Design review of the part built by this model. Coordinates are the model's own, in mm. Face numbers are marked on the shaded views. A direction names the side the tool comes from. Give positions to 0.01 mm unless a question says otherwise; leave off trailing zeros. Loops run counter-clockwise (first coordinate to the right, second up) from the corner with the lowest first, then second, coordinate; pieces in that order, holes last. Notation, with made-up numbers: (63, -16) -> (87, -16) arc R32 ccw to (87, 16) -> close; hole circle Ø10 at (-18, 18.25). An arc over 180 degrees is marked (long way). Answer in a Markdown table with one row per item. Add a question column.
(1) Consider section B-B on x = 12.5. Write out the cut boundary in (y, z), then the cut area to 3 significant figures.
(2) Draft analysis for pull direction Y (two halves, no side actions). For the marked faces 1, 2 and 3, state which applies: +Y half, -Y half, draft (parallel to the pull), parting line (faces both ways), or undercut.
(3) For line 1 (X direction, y = 25.5, z = -0.4); line 2 (Y direction, x = -12.5, z = 1.3); line 3 (X direction, y = -17.5, z = -0.25), list the stretches that pass through material, from the lowest coordinate up.
(4) Consider section D-D on y = 1.5. Write out the cut boundary in (x, z), then the cut area to 3 significant figures.
(5) For pin 1 (5 mm diameter, centred on x = -12.5, y = -12.5, fed in from -Z); pin 2 (2 mm diameter, centred on x = -2.5, z = 2, fed in from +Y); pin 3 (1.5 mm diameter, centred on y = 4.5, z = 2.5, fed in from -X), all flat-tipped, find the tip position at first contact; note any pin that passes through.
(6) Consider section A-A on x = -0.5. Write out the cut boundary in (y, z).
(7) For the marked faces 4 and 5, list the 3-axis set-ups (+Z, -Z, +X, -X, +Y, -Y) from which the entire face can be reached by the end or side of a thin tool; tool diameter is ignored.
(8) Consider section C-C on z = -3.25. Write out the cut boundary in (x, y).
from build123d import *

# Parameters (mm, degrees)
F0_R     = 1.6
F0_W     = 12
F0_H     = 15
F1_DEPTH = 4
F2_R     = 2.25
F3_DEPTH = 1
F4_DEPTH = 5
F5_R     = 5


# Not quite as in the source:
# - ends of sketch curves that miss each other by under 0.0002 mm in the source are joined


with BuildPart() as f1:
    # F0 (on Top) → F1 (new body)
    with BuildSketch(Plane.XY):
        Polygon((-26.600003, -29.899997), (-26.5, -30), (-10, -30), (10, -30), (26.5, -30), (26.6, -29.9), (27, -29.5), (27, -13), (27, 13), (27, 29.5), (26.5999975, 29.9000025), (26.5, 30), (10, 30), (-10, 30), (-26.5, 30), (-26.599999, 29.900001), (-27, 29.5), (-27, 13), (-27, -13), (-27, -29.5), align=None)
        with BuildLine():
            ThreePointArc((-22.5, -23.25), (-20.9090097423, -23.9090097423), (-20.25, -25.5))
            ThreePointArc((-20.25, -25.5), (-20.9090097423, -27.0909902577), (-22.5, -27.75))
            ThreePointArc((-22.5, -27.75), (-24.0909902577, -27.0909902577), (-24.75, -25.5))
            ThreePointArc((-24.75, -25.5), (-24.0909902577, -23.9090097423), (-22.5, -23.25))
        make_face(mode=Mode.SUBTRACT)
        with Locations((-12.5, -12.5)):
            Circle(F0_R, mode=Mode.SUBTRACT)
        with BuildLine():
            ThreePointArc((22.5, -23.25), (24.0909902577, -23.9090097423), (24.75, -25.5))
            ThreePointArc((24.75, -25.5), (24.0909902577, -27.0909902577), (22.5, -27.75))
            ThreePointArc((22.5, -27.75), (20.9090097423, -27.0909902577), (20.25, -25.5))
            ThreePointArc((20.25, -25.5), (20.9090097423, -23.9090097423), (22.5, -23.25))
        make_face(mode=Mode.SUBTRACT)
        with Locations((12.5, -12.5)):
            Circle(F0_R, mode=Mode.SUBTRACT)
        with Locations((-12.5, 12.5)):
            Circle(F0_R, mode=Mode.SUBTRACT)
        with BuildLine():
            ThreePointArc((-22.5, 27.75), (-20.9090097423, 27.0909902577), (-20.25, 25.5))
            ThreePointArc((-20.25, 25.5), (-20.9090097423, 23.9090097423), (-22.5, 23.25))
            ThreePointArc((-22.5, 23.25), (-24.0909902577, 23.9090097423), (-24.75, 25.5))
            ThreePointArc((-24.75, 25.5), (-24.0909902577, 27.0909902577), (-22.5, 27.75))
        make_face(mode=Mode.SUBTRACT)
        Rectangle(F0_W, F0_H, mode=Mode.SUBTRACT)
        with Locations((12.5, 12.5)):
            Circle(F0_R, mode=Mode.SUBTRACT)
        with BuildLine():
            ThreePointArc((22.5, 27.75), (24.0909902577, 27.0909902577), (24.75, 25.5))
            ThreePointArc((24.75, 25.5), (24.0909902577, 23.9090097423), (22.5, 23.25))
            ThreePointArc((22.5, 23.25), (20.9090097423, 23.9090097423), (20.25, 25.5))
            ThreePointArc((20.25, 25.5), (20.9090097423, 27.0909902577), (22.5, 27.75))
        make_face(mode=Mode.SUBTRACT)
        Polygon((-10, -30), (-26.5, -30), (-26.6, -30), (-27, -30), (-27, -29.5), (-27, -13), (-30, -13), (-30, -33), (-10, -33), align=None)
        Polygon((26.5, -30), (10, -30), (10, -33), (30, -33), (30, -13), (27, -13), (27, -29.5), (27, -30), (26.6, -30), align=None)
        Polygon((27, 29.5), (27, 13), (30, 13), (30, 33), (10, 33), (10, 30), (26.5, 30), (26.6, 30), (27, 30), align=None)
        Polygon((-30, 13), (-27, 13), (-27, 29.5), (-27, 30), (-26.6, 30), (-26.5, 30), (-10, 30), (-10, 33), (-30, 33), align=None)
    extrude(amount=F1_DEPTH)

    # F2 (on face) → F3 (join)
    with BuildSketch(Plane(origin=(0, 0, 0), x_dir=(1, 0, 0), z_dir=(0, 0, -1))):
        Polygon((-16.5, -30), (-16.5, 30), (-26.5, 30), (-27, 29.5), (-27, 13), (-27, -13), (-27, -29.500004), (-26.5, -30), align=None)
        with Locations((-22.5, -25.5)):
            Circle(F2_R, mode=Mode.SUBTRACT)
        with Locations((-22.5, 25.5)):
            Circle(F2_R, mode=Mode.SUBTRACT)
        Polygon((27, -13), (27, 13), (27, 29.5), (26.5, 30), (16.5, 30), (16.5, -30), (26.5, -30), (27, -29.500004), align=None)
        with Locations((22.5, -25.5)):
            Circle(F2_R, mode=Mode.SUBTRACT)
        with Locations((22.5, 25.5)):
            Circle(F2_R, mode=Mode.SUBTRACT)
    extrude(amount=F3_DEPTH)

    # F2 (on face) + F0 (on Top) → F4 (join)
    with BuildSketch(Plane(origin=(0, 0, 0), x_dir=(1, 0, 0), z_dir=(0, 0, -1))):
        Polygon((-30, 13), (-27.4, 13), (-27.4, 30.4), (-10, 30.4), (-10, 33), (-30, 33), align=None)
        Polygon((-27.4, -30.4), (-27.4, -13), (-30, -13), (-30, -33), (-10, -33), (-10, -30.4), align=None)
        Polygon((27.4, -30.4), (10, -30.4), (10, -33), (30, -33), (30, -13), (27.4, -13), align=None)
    with BuildSketch(Plane.XY):
        Polygon((26.5, -30), (10, -30), (10, -33), (30, -33), (30, -13), (27, -13), (27, -29.5), (27, -30), (26.6, -30), align=None)
    extrude(amount=F4_DEPTH, dir=(0, 0, -1))

    # F5
    f5_edges = [f1.edges().sort_by_distance(p)[0] for p in [
        (30, -33, -0.5),
        (30, 33, -0.5),
        (-30, 33, -0.5),
        (-30, -33, -0.5),
    ]]
    fillet(f5_edges, radius=F5_R)


solid = f1.part
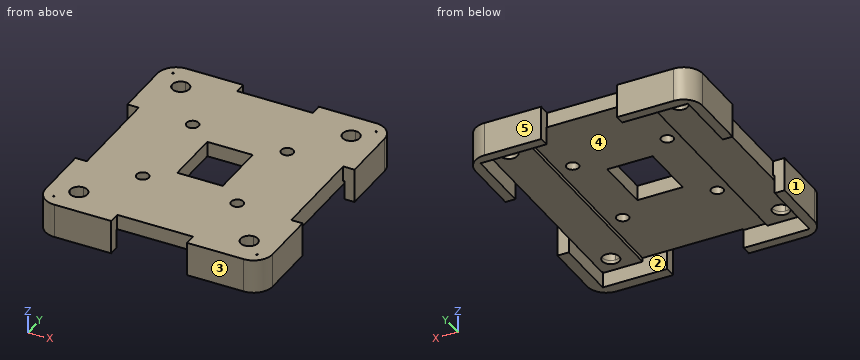
Values follow:
| question | item | result |
|---|---|---|
| 1 | outline | (-33, -5) -> (-30, -5) -> (-30, 0) -> (-14.1, 0) -> (-14.1, 4) -> (-33, 4) -> close; (-10.9, 0) -> (10.9, 0) -> (10.9, 4) -> (-10.9, 4) -> close; (14.1, 0) -> (30.4, 0) -> (30.4, -5) -> (33, -5) -> (33, 4) -> (14.1, 4) -> close |
| 1 | area | 266 mm2 |
| 2 | face 1 | draft |
| 2 | face 2 | undercut |
| 2 | face 3 | -Y half |
| 3 | line 1 | -30 to -27.4, -27 to -24.75, -20.25 to -16.5, 16.5 to 20.25, 24.75 to 27, 27.4 to 30 |
| 3 | line 2 | -33 to -14.1, -10.9 to 10.9, 14.1 to 33 |
| 3 | line 3 | -30 to -27.4, -27 to -16.5, 16.5 to 30 |
| 4 | outline | (-27, -1) -> (-16.5, -1) -> (-16.5, 0) -> (-6, 0) -> (-6, 4) -> (-27, 4) -> close; (6, 0) -> (16.5, 0) -> (16.5, -1) -> (27, -1) -> (27, 4) -> (6, 4) -> close |
| 4 | area | 189 mm2 |
| 5 | pin 1 | z = 0 |
| 5 | pin 2 | y = 30 |
| 5 | pin 3 | x = -27 |
| 6 | outline | (-30, 0) -> (-7.5, 0) -> (-7.5, 4) -> (-30, 4) -> close; (7.5, 0) -> (30, 0) -> (30, 4) -> (7.5, 4) -> close |
| 7 | face 4 | -Z |
| 7 | face 5 | +Z, -Z, +X, -X, +Y |
| 8 | outline | (-30, -28) arc R5 ccw to (-25, -33) -> (-10, -33) -> (-10, -30.4) -> (-27.4, -30.4) -> (-27.4, -13) -> (-30, -13) -> close; (-30, 13) -> (-27.4, 13) -> (-27.4, 30.4) -> (-10, 30.4) -> (-10, 33) -> (-25, 33) arc R5 ccw to (-30, 28) -> close; (10, -33) -> (25, -33) arc R5 ccw to (30, -28) -> (30, -13) -> (27, -13) -> (27, -30) -> (10, -30) -> close; (10, 30.4) -> (27.4, 30.4) -> (27.4, 13) -> (30, 13) -> (30, 28) arc R5 ccw to (25, 33) -> (10, 33) -> close |
